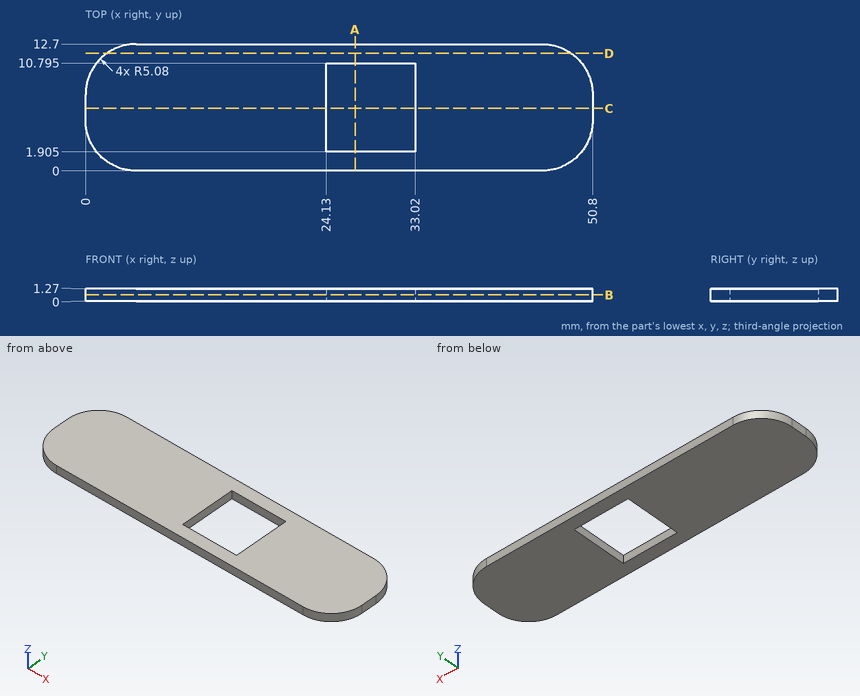
Part print with two shaded views. Sizes in mm from the minimum x, y, z corner. Coordinates: 2 decimals unless noted, no trailing zeros. Write each loop counter-clockwise with the first axis right and the second up, starting at its lowest first coordinate (ties: lowest second). Pieces come first, ordered by that corner, then holes.
1. Band-saw the part on A-A, the plane x = 27. Give the cut face in (y, z) (3 decimals), and give its area (3 significant figures).
Answer block:
outline: (0, 0) - (1.905, 0) - (1.905, 1.27) - (0, 1.27) - close; (10.795, 0) - (12.7, 0) - (12.7, 1.27) - (10.795, 1.27) - close
area: 4.84 mm2
2. Drill centre lines: probe 1 along X at (y, z) = (6, 0.65); probe 2 along Y at (x, z) = (31, 0.75) (3 decimals); probe 3 along X at (y, z) = (2.25, 0.4). Where is each one in solid material? Low to high.
Answer block:
probe 1: x = 0 to 24.13, 33.02 to 50.8
probe 2: y = 0 to 1.905, 10.795 to 12.7
probe 3: x = 0.86 to 24.13, 33.02 to 49.94
3. Band-saw the part on B-B, the plane z = 0.65. Give the cut face in (x, y) (3 decimals).
Answer block:
outline: (0, 5.08) arc R5.08 ccw to (5.08, 0) - (45.72, 0) arc R5.08 ccw to (50.8, 5.08) - (50.8, 7.62) arc R5.08 ccw to (45.72, 12.7) - (5.08, 12.7) arc R5.08 ccw to (0, 7.62) - close; hole (24.13, 1.905) - (33.02, 1.905) - (33.02, 10.795) - (24.13, 10.795) - close
4. Band-saw the part on D-D, the plane y = 11.75. Give the cut face in (x, z), and give its area (3 significant figures).
Answer block:
outline: (2.12, 0) - (48.68, 0) - (48.68, 1.27) - (2.12, 1.27) - close
area: 59.1 mm2
5. Band-saw the part on C-C, the plane y = 6.25. Give the cut face in (x, z), and give its area (3 significant figures).
Answer block:
outline: (0, 0) - (24.13, 0) - (24.13, 1.27) - (0, 1.27) - close; (33.02, 0) - (50.8, 0) - (50.8, 1.27) - (33.02, 1.27) - close
area: 53.2 mm2
